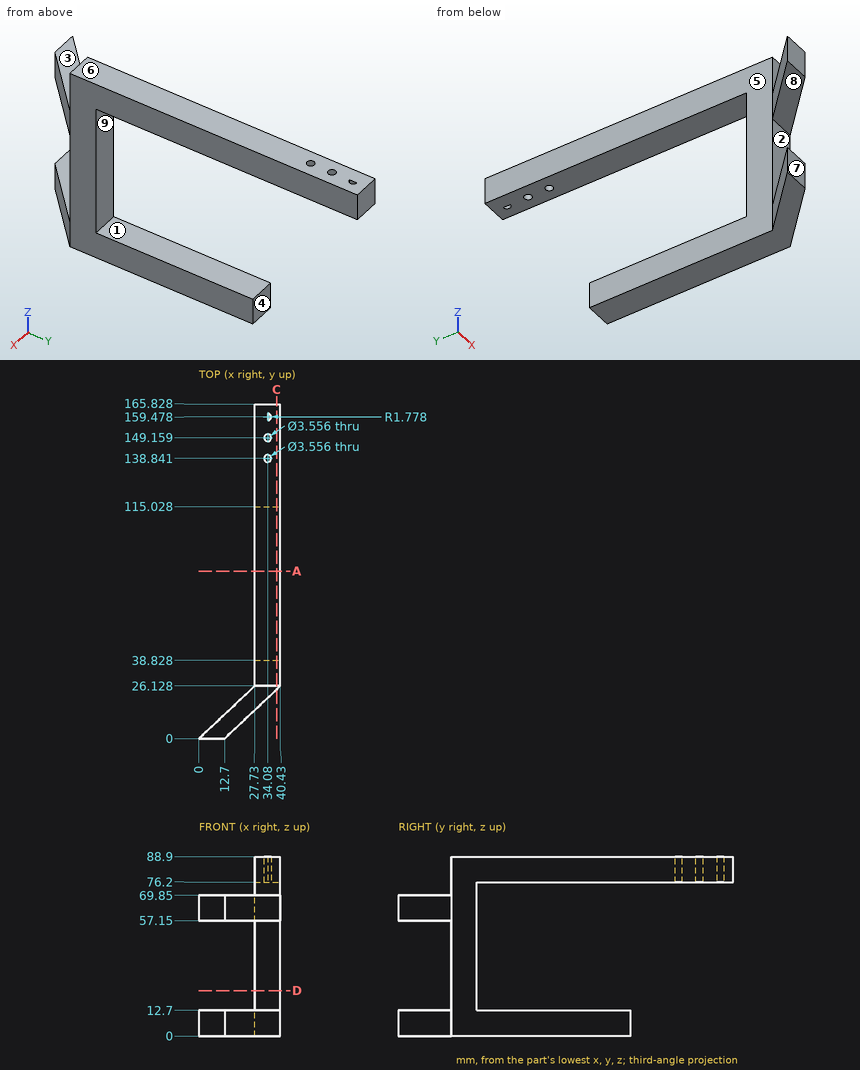
Drawing for the job (mm, zero at the part's lowest x, y, z). A direction names the side the tool comes from. Round coordinates to 2 decimals unless told otherwise and drop trailing zeros. Order: outer loops, then holes, each group sorted by start corner. A loop starts at its lowest first (then second) coordinate and runs counter-clockwise, first axis right, second up. Notation, with made-up numbers: (36, 33.25) -> (56, 33.25) arc R22 ccw to (56, 56.25) -> close; hole circle Ø6 at (-30, -30). An arc over 180 degrees is marked (long way). Put each result on its own line as item: value.
Q1. Pull direction Z, two halves, no side cores. Call the marked faces 6, 7, 8 and 9: pulls with the +Z half, pulls with the -Z half, needs draft (parallel to the pull), parting line crosses it, or undercut.
From the geometry:
face 6: pulls with the +Z half
face 7: needs draft
face 8: undercut
face 9: undercut
Q2. Pin check, flat tips, straight feed: pin 1 Ø6.5 at (x, z) = (36.5, 59) entering from +Y; pin 2 Ø13 at (x, y) = (17.5, 9.5) entering from +Z; pin 3 Ø4 at (x, z) = (33.5, 78) entering from -Y. Stop position of each tip, or through.
From the geometry:
pin 1: stops at y = 38.83
pin 2: stops at z = 69.85
pin 3: stops at y = 26.13
Q3. Band-saw the part on A-A (y = 83). Give the cut face in (x, z).
From the geometry:
outline: (27.73, 0) -> (40.43, 0) -> (40.43, 12.7) -> (27.73, 12.7) -> close; (27.73, 76.2) -> (40.43, 76.2) -> (40.43, 88.9) -> (27.73, 88.9) -> close
Q4. Tool access for the marked faces 1, 2, 3, 4 and 5: list every direction of +Z, -Z, +X, -X, +Y, -Y with a clear straight run to the whole face (end or side of a thin tool).
From the geometry:
face 1: +X, -X, +Y
face 2: +X, -X, -Y
face 3: +Z, +X, -X, -Y
face 4: -Z, +X, -X, +Y
face 5: +Z, -Z, -X, +Y
Q5. Band-saw the part on C-C (x = 38.5). Give the cut face in (y, z).
From the geometry:
outline: (24.31, 0) -> (115.03, 0) -> (115.03, 12.7) -> (38.83, 12.7) -> (38.83, 76.2) -> (165.83, 76.2) -> (165.83, 88.9) -> (26.13, 88.9) -> (26.13, 69.85) -> (24.31, 69.85) -> (24.31, 57.15) -> (26.13, 57.15) -> (26.13, 12.7) -> (24.31, 12.7) -> close
Q6. Wall check: line 1 (Z direction, x = 29.5, y = 82.5); line 2 (Y direction, x = 39, z = 15.5); line 3 (X direction, y = 159, z = 85.5). Give the ranges that are in metal, low to high. Write a range as [from, to].
From the geometry:
line 1: z = [0, 12.7], [76.2, 88.9]
line 2: y = [26.13, 38.83]
line 3: x = [27.73, 34.08], [35.79, 40.43]
Q7. Band-saw the part on D-D (z = 22.5). Give the cut face in (x, y), and give its area (3 significant figures).
From the geometry:
outline: (27.73, 26.13) -> (40.43, 26.13) -> (40.43, 38.83) -> (27.73, 38.83) -> close
area: 161 mm2
